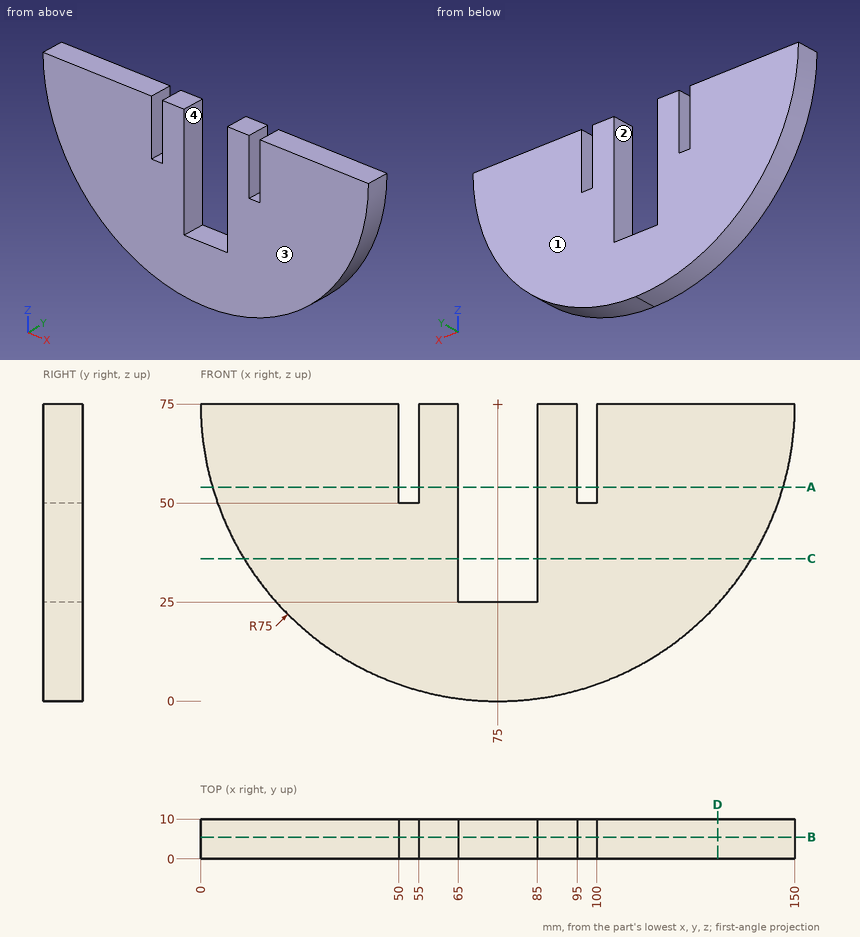
Verification items for this drawing (mm, ordinates from the low corner). A direction names the side the tool comes from. Give positions to 0.01 mm unless a question says otherwise; leave off trailing zeros. Order: outer loops, then holes, each group sorted by start corner. A loop starts at its lowest first (then second) coordinate and runs counter-clockwise, first axis right, second up. Notation, with made-up numbers: M -5,62.25 L 0,62.25 A25 cw 0,76.25 Z; hole C 87,53 d1. An arc over 180 degrees is marked long. Use a Markdown table: item, result.
Item 1: Depth check by flat-ended pin: P1, Ø4, axis at x = 52.5, y = 2, coming from the -Z side; P2, Ø5, axis at y = 5.5, z = 61, coming from the +X side; P3, Ø3, axis at x = 79, y = 3.5, coming from the +Z side. Enter the tip coordinate at first touch or a pass-through.
Answers follow:
| item | result |
|---|---|
| P1 | stops at z = 2.86 |
| P2 | stops at x = 149.11 |
| P3 | stops at z = 25 |
Item 2: Tool access check on the marked faces 3 and 4. Record the directions out of +Z, -Z, +X, -X, +Y, -Y that give a thin tool (end or side, any length) a straight path to the whole face; none if there is none.
Answers follow:
| item | result |
|---|---|
| face 3 | +Z, -Z, +X, -X, -Y |
| face 4 | +Z, +Y, -Y |
Item 3: Section check B-B (y = 5.5). Record the cut outline in (x, z), and give its area (3 significant figures).
Answers follow:
| item | result |
|---|---|
| outline | M 0,75 A75 ccw 75,0 A75 ccw 150,75 L 100,75 L 100,50 L 95,50 L 95,75 L 85,75 L 85,25 L 65,25 L 65,75 L 55,75 L 55,50 L 50,50 L 50,75 Z |
| area | 7,590 mm2 |
Item 4: Section check C-C (z = 36). Record the cut outline in (x, y), and give its area (3 significant figures).
Answers follow:
| item | result |
|---|---|
| outline | M 10.94,0 L 65,0 L 65,10 L 10.94,10 Z; M 85,0 L 139.06,0 L 139.06,10 L 85,10 Z |
| area | 1,080 mm2 |
Item 5: Section check A-A (z = 54). Record the cut outline in (x, y), and give its area (3 significant figures).
Answers follow:
| item | result |
|---|---|
| outline | M 3,0 L 50,0 L 50,10 L 3,10 Z; M 55,0 L 65,0 L 65,10 L 55,10 Z; M 85,0 L 95,0 L 95,10 L 85,10 Z; M 100,0 L 147,0 L 147,10 L 100,10 Z |
| area | 1,140 mm2 |
Item 6: Material ranges on line 1 along X through (y, z) = (0.5, 61); line 2 along X through (y, z) = (9.5, 46.5); line 3 along X through (y, z) = (6.75, 30), recorded low to high.
Answers follow:
| item | result |
|---|---|
| line 1 | x = 1.32 to 50, 55 to 65, 85 to 95, 100 to 148.68 |
| line 2 | x = 5.63 to 65, 85 to 144.37 |
| line 3 | x = 15 to 65, 85 to 135 |
Item 7: Draft check along X on the marked faces 1 and 2. Enter one of: +X half, -X half, draft (parallel to the pull), parting line (faces both ways), or undercut.
Answers follow:
| item | result |
|---|---|
| face 1 | draft |
| face 2 | undercut |
Item 8: Section check D-D (x = 130.5). Record the cut outline in (y, z), and give its area (3 significant figures).
Answers follow:
| item | result |
|---|---|
| outline | M 0,24.55 L 10,24.55 L 10,75 L 0,75 Z |
| area | 504 mm2 |
